Part model, mm, in its own coordinate system. Give positions to 0.01 mm unless a question says otherwise; leave off trailing zeros. Order: outer loops, then holes, each group sorted by start corner. A loop starts at its lowest first (then second) coordinate and runs counter-clockwise, first axis right, second up. Notation, with made-up numbers: (-5, 78.25) -> (24, 78.25) arc R17 ccw to (24, 94.25) -> close; hole circle Ø3 at (71.25, 82). An arc over 180 degrees is marked (long way). Write item = value, one per line. Start each with the question number.
(1) Saw through at A-A, the plane y = 0. List the corners of the cut face in (x, z).
(2) Probe line 1 along Y through (x, z) = (0, 0.45); line 2 along Y through (x, z) = (1.5, 0.25); line 3 along X through (y, z) = (3.5, 0.1). List the from-to ranges inside material, lowest first. Write a range as from..to.
(3) Saw through at B-B, the plane x = -1.5. List the corners of the cut face in (y, z).
(4) Saw through at D-D, the plane y = -3. List the corners of the cut face in (x, z).
(5) Saw through at C-C, the plane z = 0.7. List the corners of the cut face in (x, y), then the cut area to 3 significant figures.
(6) Flat gauge pins, fed straight in: pin 1 (1.5 mm diameter, centred on x = -1, y = 3.5, fed in from -Z); pin 2 (3 mm diameter, centred on x = 0, y = 0, fed in from -Z). Where does each tip first touch, or does it go through?
Autodesk Inventor part; units mm, degrees
ref_plane "YZ Plane" through (0, 0, 0) normal (1, 0, 0) x (0, 1, 0)
ref_plane "XZ Plane" through (0, 0, 0) normal (0, 1, 0) x (-1, 0, 0)
ref_plane "XY Plane" through (0, 0, 0) normal (0, 0, 1) x (1, 0, 0)
sketch "Эскиз1" plane through (0, 0, 0) normal (0, 0, 1) x (1, 0, 0)
  circle A0 centre (0, 0) radius 4.5
  dimension "d0" = 9
extrude "Выдавливание1" add sketch "Эскиз1" along normal blind 0.8
sketch "Эскиз2" plane through (0, 0, 0.8) normal (0, 0, 1) x (1, 0, 0)
  circle A0 centre (0, 0) radius 1.8
  dimension "d3" = 3.6
extrude "Выдавливание2" cut sketch "Эскиз2" against normal blind 0.8
sketch "Эскиз3" plane through (0, 0, 0.8) normal (0, 0, 1) x (1, 0, 0)
  line L0 (0, 0) -> (0, -3.5)
  line L1 (0, 0) -> (-4, 0)
  circle A0 centre (0, 0) radius 4.5
  line L2 (-4, -2.0616) -> (-5.2131, -2.0616)
  line L3 (-5.2131, -2.0616) -> (-5.2131, 3.1786)
  line L4 (-5.2131, 3.1786) -> (-4, 3.1786)
  line L5 (-4, 3.1786) -> (-4, -2.0616)
  line L6 (-2.8284, -3.5) -> (4.77, -3.5)
  line L7 (4.77, -3.5) -> (4.77, -5.6057)
  line L8 (4.77, -5.6057) -> (-2.8284, -5.6057)
  line L9 (-2.8284, -5.6057) -> (-2.8284, -3.5)
  dimension "d6" = 3.5
  dimension "d7" = 4
extrude "Выдавливание3" cut sketch "Эскиз3" against normal blind 10 contours L6 A0 | L5 A0 | A0 L6 L7 L8 L9 | L2 L3 L4 L5 A0
properties part number "shayba"
Results list:
q1.outline = (-4, 0) -> (-1.8, 0) -> (-1.8, 0.8) -> (-4, 0.8) -> close; (1.8, 0) -> (4.5, 0) -> (4.5, 0.8) -> (1.8, 0.8) -> close
q2.line_1 = -3.5..-1.8, 1.8..4.5
q2.line_2 = -3.5..-0.99, 0.99..4.24
q2.line_3 = -2.83..2.83
q3.outline = (-3.5, 0) -> (-0.99, 0) -> (-0.99, 0.8) -> (-3.5, 0.8) -> close; (0.99, 0) -> (4.24, 0) -> (4.24, 0.8) -> (0.99, 0.8) -> close
q4.outline = (-3.35, 0) -> (3.35, 0) -> (3.35, 0.8) -> (-3.35, 0.8) -> close
q5.outline = (-4, -2.06) arc R4.5 ccw to (-2.83, -3.5) -> (2.83, -3.5) arc R4.5 ccw (long way) to (-4, 2.06) -> close; hole circle Ø3.6 at (0, 0)
q5.area = 48.2 mm^2
q6.pin_1 = 0
q6.pin_2 = through
